from build123d import *

# Parameters (mm, degrees)
SKETCH1_R           = 1.675
BOSS_EXTRUDE1_DEPTH = 2
SKETCH2_W           = 49.5
SKETCH2_H           = 37.5
SKETCH2_R           = 1.6
BOSS_EXTRUDE2_DEPTH = 2
FILLET1_R           = 2.5
FILLET2_R           = 1


with BuildPart() as part:
    # Sketch1 → Boss-Extrude1 (new body)
    with BuildSketch(Plane(origin=(0, 0, 0), x_dir=(0, 0, -1), z_dir=(1, 0, 0))):
        with BuildLine():
            Line((-18.75, 0), (18.75, 0))
            Line((18.75, 0), (18.75, 20.85))
            ThreePointArc((18.75, 20.85), (0, 39.6), (-18.75, 20.85))
            Line((-18.75, 20.85), (-18.75, 0))
        make_face()
        with Locations((-7.825, 7.296702431)):
            Circle(SKETCH1_R, mode=Mode.SUBTRACT)
        with Locations((7.825, 7.296702431)):
            Circle(SKETCH1_R, mode=Mode.SUBTRACT)
        with Locations((-15.65, 20.85)):
            Circle(SKETCH1_R, mode=Mode.SUBTRACT)
        with Locations((-7.825, 34.403297569)):
            Circle(SKETCH1_R, mode=Mode.SUBTRACT)
        with BuildLine():
            Line((-6.565, 12.35), (-6.565, 29.35))
            ThreePointArc((-6.565, 29.35), (0, 35.915), (6.565, 29.35))
            Line((6.565, 29.35), (6.565, 12.35))
            ThreePointArc((6.565, 12.35), (0, 5.785), (-6.565, 12.35))
        make_face(mode=Mode.SUBTRACT)
        with Locations((15.65, 20.85)):
            Circle(SKETCH1_R, mode=Mode.SUBTRACT)
        with Locations((7.825, 34.403297569)):
            Circle(SKETCH1_R, mode=Mode.SUBTRACT)
    extrude(amount=BOSS_EXTRUDE1_DEPTH)

    # Sketch2 → Boss-Extrude2 (add)
    with BuildSketch(Plane(origin=(0, 0, 0), x_dir=(1, 0, 0), z_dir=(0, 1, 0))):
        with Locations((-24.75, 0)):
            Rectangle(SKETCH2_W, SKETCH2_H)
        with Locations((-44.9875, 15.75)):
            Circle(SKETCH2_R, mode=Mode.SUBTRACT)
        with Locations((-38.6, 15.75)):
            Circle(SKETCH2_R, mode=Mode.SUBTRACT)
        with Locations((-32.2125, 15.75)):
            Circle(SKETCH2_R, mode=Mode.SUBTRACT)
        with Locations((-25.825, 15.75)):
            Circle(SKETCH2_R, mode=Mode.SUBTRACT)
        with Locations((-19.4375, 15.75)):
            Circle(SKETCH2_R, mode=Mode.SUBTRACT)
        with Locations((-13.05, 15.75)):
            Circle(SKETCH2_R, mode=Mode.SUBTRACT)
        with Locations((-6.6625, 15.75)):
            Circle(SKETCH2_R, mode=Mode.SUBTRACT)
        with Locations((-6.6625, -15.75)):
            Circle(SKETCH2_R, mode=Mode.SUBTRACT)
        with Locations((-13.05, -15.75)):
            Circle(SKETCH2_R, mode=Mode.SUBTRACT)
        with Locations((-19.4375, -15.75)):
            Circle(SKETCH2_R, mode=Mode.SUBTRACT)
        with Locations((-44.9875, -15.75)):
            Circle(SKETCH2_R, mode=Mode.SUBTRACT)
        with Locations((-38.6, -15.75)):
            Circle(SKETCH2_R, mode=Mode.SUBTRACT)
        with Locations((-32.2125, -15.75)):
            Circle(SKETCH2_R, mode=Mode.SUBTRACT)
        with Locations((-25.825, -15.75)):
            Circle(SKETCH2_R, mode=Mode.SUBTRACT)
    extrude(amount=BOSS_EXTRUDE2_DEPTH)

    # Fillet1
    fillet1_edges = [part.edges().sort_by_distance(p)[0] for p in [
        (-49.5, 1, 18.75),
        (-49.5, 1, -18.75),
        (2, 0, 0),
    ]]
    fillet(fillet1_edges, radius=FILLET1_R)

    # Fillet2
    fillet2_edges = [part.edges().sort_by_distance(p)[0] for p in [
        (0, 2, 0),
    ]]
    fillet(fillet2_edges, radius=FILLET2_R)


solid = part.part
Geometry check sheet. Reference: the model listing, model coordinates, mm. Coordinates: 2 decimals unless noted, no trailing zeros. Write each loop counter-clockwise with the first axis right and the second up, starting at its lowest first coordinate (ties: lowest second). Pieces come first, ordered by that corner, then holes. Notation, with made-up numbers: (-10, 76.25) -> (45, 76.25) arc R10 cw to (45, 86.25) -> close; hole circle Ø1 at (-23.5, 45). An arc over 180 degrees is marked (long way). One line per question, with ' | ' between items.
1. Thickness scan on probe 1 along X at (y, z) = (3, -16). Record the ranges inside material, lowest first. Write a range as from..to.
Answers:
probe 1: x = 0..2
2. Cross-section at C-C on y = 4. Record the cut outline in (x, z), and give its area (3 significant figures).
Answers:
outline: (0, -18.75) -> (2, -18.75) -> (2, 18.75) -> (0, 18.75) -> close | area: 75.0 mm²
3. Cross-section at A-A on z = 0. Record the cut outline in (x, y) (3 decimals), and give its area (3 significant figures).
Answers:
outline: (-49.5, 0) -> (-0.5, 0) arc R2.5 ccw to (2, 2.5) -> (2, 5.785) -> (0, 5.785) -> (0, 3) arc R1 cw to (-1, 2) -> (-49.5, 2) -> close; (0, 35.915) -> (2, 35.915) -> (2, 39.6) -> (0, 39.6) -> close | area: 117 mm²
4. Cross-section at B-B on x = -19. Record the cut outline in (y, z), and give its area (3 significant figures).
Answers:
outline: (0, -18.75) -> (2, -18.75) -> (2, -17.29) -> (0, -17.29) -> close; (0, -14.21) -> (2, -14.21) -> (2, 14.21) -> (0, 14.21) -> close; (0, 17.29) -> (2, 17.29) -> (2, 18.75) -> (0, 18.75) -> close | area: 62.7 mm²
5. Depth check by flat-ended pin: pin 1 Ø4 at (x, z) = (-7.5, -8) entering from +Y; pin 2 Ø1.9 at (x, z) = (-25.825, 15.75) entering from -Y; pin 3 Ø2 at (x, y) = (1.5, 24.5) entering from -Z; pin 4 Ø3 at (y, z) = (17.5, -6.5) entering from -X. Enter the tip coordinate at first touch or a pass-through.
Answers:
pin 1: stops at y = 2 | pin 2: passes through | pin 3: stops at z = -18.56 | pin 4: stops at x = 0
6. Cross-section at D-D on z = -13. Record the cut outline in (x, y).
Answers:
outline: (-49.5, 0) -> (-0.5, 0) arc R2.5 ccw to (2, 2.5) -> (2, 34.36) -> (0, 34.36) -> (0, 3) arc R1 cw to (-1, 2) -> (-49.5, 2) -> close
7. Draft check along X on faces 1 (the cylindrical face through (-46.586, 0.986, 15.68)), 2 (the flat face through (0, 17, -8)), 3 (the cylindrical face through (-46.586, 0.986, -15.82)), 4 (the flat face through (1, 21, -6.565)). Enter one of: +X half, -X half, draft (parallel to the pull), parting line (faces both ways), or undercut.
Answers:
face 1: undercut | face 2: -X half | face 3: undercut | face 4: draft
